Input: part model. Units: mm. Frame: model coordinates. A direction names the side the tool comes from. Coordinates: 2 decimals unless noted, no trailing zeros. Order: outer loops, then holes, each group sorted by start corner. A loop starts at its lowest first (then second) coordinate and runs counter-clockwise, first axis right, second up.
from build123d import *

# Parameters (mm, degrees)
SKETCH2_R   = 7.874
SKETCH2_R_2 = 6.35


with BuildPart() as part:
    # Sweep1: sweep along a path in Sketch1
    with BuildLine(Plane.XY) as sweep1_path:
        Line((28.068079684, 0), (0, 0))
        ThreePointArc((0, 0), (-9.946095847, -0.651901563), (-19.722011237, -2.596452037))
        Line((-19.722011237, -2.596452037), (-50.523992361, -10.849818004))
        ThreePointArc((-50.523992361, -10.849818004), (-60.299907751, -12.794368478), (-70.246003598, -13.446270041))
        Line((-70.246003598, -13.446270041), (-98.314083282, -13.446270041))
    # Sketch2 → Sweep1 (sweep)
    with BuildSketch(Plane.ZY.offset(-28.068079684)):
        Circle(SKETCH2_R)
        Circle(SKETCH2_R_2, mode=Mode.SUBTRACT)
    sweep(path=sweep1_path.line)


solid = part.part
Item 1: Cut plane A-A on z = 0. Return loops of the section in (x, y), then the cut area to 3 significant figures.
Response values:
outline: (-98.31, -21.32) - (-70.25, -21.32) arc R84.07 ccw to (-48.49, -18.46) - (-17.68, -10.2) arc R68.33 cw to (0, -7.87) - (28.07, -7.87) - (28.07, -6.35) - (0, -6.35) arc R69.85 ccw to (-18.08, -8.73) - (-48.88, -16.98) arc R82.55 cw to (-70.25, -19.8) - (-98.31, -19.8) - close; (-98.31, -7.1) - (-70.25, -7.1) arc R69.85 ccw to (-52.17, -4.72) - (-21.37, 3.54) arc R82.55 cw to (0, 6.35) - (28.07, 6.35) - (28.07, 7.87) - (0, 7.87) arc R84.07 ccw to (-21.76, 5.01) - (-52.56, -3.24) arc R68.33 cw to (-70.25, -5.57) - (-98.31, -5.57) - close
area: 390 mm2
Item 2: Cut plane C-C on z = 4.75. Return loops of the section in (x, y).
Response values:
outline: (-98.31, -19.73) - (-70.25, -19.73) arc R82.48 ccw to (-48.9, -16.92) - (-18.1, -8.66) arc R69.92 cw to (0, -6.28) - (28.07, -6.28) - (28.07, -4.21) - (0, -4.21) arc R71.99 ccw to (-18.63, -6.67) - (-49.43, -14.92) arc R80.41 cw to (-70.25, -17.66) - (-98.31, -17.66) - close; (-98.31, -9.23) - (-70.25, -9.23) arc R71.99 ccw to (-51.61, -6.78) - (-20.81, 1.47) arc R80.41 cw to (0, 4.21) - (28.07, 4.21) - (28.07, 6.28) - (0, 6.28) arc R82.48 ccw to (-21.35, 3.47) - (-52.15, -4.78) arc R69.92 cw to (-70.25, -7.17) - (-98.31, -7.17) - close
Item 3: Cut plane B-B on x = 5.5. Return loops of the section in (y, z), then the cut area to 3 significant figures.
Response values:
outline: circle Ø15.75 at (0, 0); hole circle Ø12.7 at (0, 0)
area: 68.1 mm2
Item 4: Pin query (flat end, axial travel): pin 1 Ø5 at (x, y) = (-63, -17) entering from +Z; pin 2 Ø1.5 at (x, z) = (-50, -1.5) entering from -Y; pin 3 Ø1 at (x, y) = (0.5, 3.5) entering from -Z. Return the tip coordinate at first contact, or that it passes through.
Response values:
pin 1: stops at z = 7.75
pin 2: stops at y = -18.92
pin 3: stops at z = -7.28
Item 5: Draft query along Z for faces 3 (the face through (13.838, -7.687, -1.707)), 4 (the face through (-33.881, -12.222, 2.93)), 5 (the face through (28.068, -6.5, -0.5)), 6 (the face through (13.84, -6.2, -1.38)). Return one class per face: pulls with the +Z half, pulls with the -Z half, needs draft (parallel to the pull), parting line crosses it, or undercut.
Response values:
face 3: parting line crosses it
face 4: undercut
face 5: needs draft
face 6: undercut
Item 6: Access query for faces 1 (the face through (-35.95, -4.5, 7.51)), 2 (the face through (-84.48, -11.08, 7.51)). Directions: +Z, -Z, +X, -X, +Y, -Y. A direction counts if a zero-diameter tool reaches every point of the face in a straight line with its end or side. Return the directions, or none.
Response values:
face 1: none
face 2: -X
Item 7: Ray query, probe 1 along Y at (x, z) = (-87.25, 0); probe 2 along Y at (x, z) = (15, 0); probe 3 along Z at (x, y) = (13, -4.75). Return the intervals inside material, ascending.
Response values:
probe 1: y = -21.32 to -19.8, -7.1 to -5.57
probe 2: y = -7.87 to -6.35, 6.35 to 7.87
probe 3: z = -6.28 to -4.21, 4.21 to 6.28
